Autodesk Inventor part; units mm, degrees
ref_plane "YZ Plane" through (0, 0, 0) normal (1, 0, 0) x (0, 1, 0)
ref_plane "XZ Plane" through (0, 0, 0) normal (0, 1, 0) x (-1, 0, 0)
ref_plane "XY Plane" through (0, 0, 0) normal (0, 0, 1) x (1, 0, 0)
sketch "スケッチ1" plane through (0, 0, 0) normal (1, 0, 0) x (0, 1, 0)
  line L0 (-11, -24) -> (11, -24)
  line L1 (11, -24) -> (11, 24)
  line L2 (11, 24) -> (-11, 24)
  line L3 (-11, 24) -> (-11, -24)
  line L4 (-11, -24) -> (11, 24) construction
  line L5 (11, -24) -> (-11, 24) construction
  point P0 (0, 0)
  dimension "d0" = 22
  dimension "d1" = 48
extrude "押し出し1" add sketch "スケッチ1" along normal blind 1.5
sketch "スケッチ2" plane through (1.5, 0, 0) normal (1, 0, 0) x (0, 0, -1)
  line L0 (-24, 11) -> (-24, -11)
  line L1 (24, -11) -> (24, 11)
  line L2 (-24, -11) -> (24, -11)
  point P0 (0, 0)
  point P1 (-20, 1)
  point P2 (20, 1)
  dimension "d4" = 4
  dimension "d5" = 4
  dimension "d6" = 12
hole "穴1" at (1.5, 1, 20) at (1.5, 1, -20) direction (-1, 0, 0) diameter 3 end through all
sketch "スケッチ3" plane through (0, 0, 0) normal (-1, 0, 0) x (0, 0, 1)
  line L0 (-5.5, -3.75) -> (8, -3.75)
  line L1 (8, -3.75) -> (8, 5.75)
  line L2 (8, 5.75) -> (-5.5, 5.75)
  line L3 (-5.5, 5.75) -> (-5.5, -3.75)
  line L4 (24, -11) -> (-24, -11)
  line L5 (-24, -11) -> (-24, 11)
  point P0 (0, 0)
  dimension "d14" = 7.25
  dimension "d15" = 18.5
  dimension "d16" = 32
  dimension "d17" = 16.75
extrude "押し出し2" cut sketch "スケッチ3" against normal blind 1.5
properties part number "sensor_pcb" material "ガラス"
The listing builds one solid part. Answer for the finished solid, in the listing's coordinates (mm). A direction names the side the tool comes from. Coordinates: 2 decimals unless noted, no trailing zeros. Loops run counter-clockwise (first coordinate to the right, second up) from the corner with the lowest first, then second, coordinate; pieces in that order, holes last. Notation, with made-up numbers: M 69,-33.5 L 121,-33.5 A30 ccw 121,4.5 Z; hole C 58.5,83 d7. An arc over 180 degrees is marked long. Answer as a JSON object with one key per item and string values. Group by question number.
Item 1: This flat-tipped pin is pushed along its axis until it touches: P1, Ø1, axis at y = -1.5, z = 2.5, coming from the -X side. Where does it stop, or does it pass through?
Item 2: Section C-C (y = 1) is taken. Write down the section's boundary in (x, z).
Item 3: Section A-A (z = 4) is taken. Write down the section's boundary in (x, y), and give its area (4 significant figures).
Item 4: Section D-D (z = -20) is taken. Write down the section's boundary in (x, y).
Item 5: Which of the six approach directions +Z, -Z, +X, -X, +Y, -Y give full straight-line access (tool end or side, diameter ignored) to faces 5 (the face through (1, -3.75, 1)), 6 (the face through (1, -11, 0))?
Item 6: Consider L1, parallel to Z at x = 0.5, y = 1; L2, parallel to Y at x = 0.5, z = -20; L3, parallel to Z at x = 0.5, y = -1.25. Determine where each line is inside the solid, lowest interval first.
Item 7: Section B-B (x = 0.9) is taken. Write down the section's boundary in (y, z).
Item 8: Determine the mould class of faces 1 (the face through (0, -5, 0)), 2 (the face through (1, 1, 8)), 3 (the face through (1, 1, -5.5)), 4 (the face through (1, 11, 0)) for opening direction Y: +Y half, -Y half, draft (parallel to the pull), parting line (faces both ways), or undercut.
Solved:
{
 "1": {"P1": "passes through"},
 "2": {"outline": "M 0,-24 L 1.5,-24 L 1.5,-21.5 L 0,-21.5 Z; M 0,-18.5 L 1.5,-18.5 L 1.5,-5.5 L 0,-5.5 Z; M 0,8 L 1.5,8 L 1.5,18.5 L 0,18.5 Z; M 0,21.5 L 1.5,21.5 L 1.5,24 L 0,24 Z"},
 "3": {"outline": "M 0,-11 L 1.5,-11 L 1.5,-3.75 L 0,-3.75 Z; M 0,5.75 L 1.5,5.75 L 1.5,11 L 0,11 Z", "area": "18.75 mm2"},
 "4": {"outline": "M 0,-11 L 1.5,-11 L 1.5,-0.5 L 0,-0.5 Z; M 0,2.5 L 1.5,2.5 L 1.5,11 L 0,11 Z"},
 "5": {"face 5": "+X, -X", "face 6": "+Z, -Z, +X, -X, -Y"},
 "6": {"L1": "z = -24 to -21.5, -18.5 to -5.5, 8 to 18.5, 21.5 to 24", "L2": "y = -11 to -0.5, 2.5 to 11", "L3": "z = -24 to -5.5, 8 to 24"},
 "7": {"outline": "M -11,-24 L 11,-24 L 11,24 L -11,24 Z; hole M -3.75,-5.5 L 5.75,-5.5 L 5.75,8 L -3.75,8 Z; hole C 1,-20 d3; hole C 1,20 d3"},
 "8": {"face 1": "draft", "face 2": "undercut", "face 3": "undercut", "face 4": "+Y half"}
}
